from build123d import *

# Parameters (mm, degrees)
SKETCH2_R         = 104.775
SKETCH2_R_2       = 67.818
FLANGE_DEPTH      = 25.4
SKETCH4_R         = 81.407
SKETCH4_R_2       = 74.295
GROOVE_DEPTH      = 3.9878
SKETCH5_R         = 2.5527
SCREW_HOLES_DEPTH = 25.4
CIRPATTERN1_COUNT = 12


with BuildPart() as part:
    # Sketch2 → Flange (new body)
    with BuildSketch(Plane(origin=(0, 0, 0), x_dir=(1, 0, 0), z_dir=(0, 1, 0))):
        with Locations(Location((0, 0, 0), (0, 0, 270))):
            Circle(SKETCH2_R)
        with Locations(Location((0, 0, 0), (0, 0, 270))):
            Circle(SKETCH2_R_2, mode=Mode.SUBTRACT)
    extrude(amount=FLANGE_DEPTH)

    # Sketch4 → Groove (cut)
    with BuildSketch(Plane(origin=(0, 25.4, 0), x_dir=(1, 0, 0), z_dir=(0, 1, 0))):
        with Locations(Location((0, 0, 0), (0, 0, 270))):
            Circle(SKETCH4_R)
        with Locations(Location((0, 0, 0), (0, 0, 270))):
            Circle(SKETCH4_R_2, mode=Mode.SUBTRACT)
    extrude(amount=-GROOVE_DEPTH, mode=Mode.SUBTRACT)

    # Sketch5 → Screw Holes (cut)
    with BuildSketch(Plane(origin=(0, 25.4, 0), x_dir=(1, 0, 0), z_dir=(0, 1, 0))):
        with Locations(Location((0, -97.25025, 0), (0, 0, 270))):
            Circle(SKETCH5_R)
    screw_holes = extrude(amount=-SCREW_HOLES_DEPTH, mode=Mode.SUBTRACT)

    # CirPattern1: Screw Holes ×12 about axis
    cirpattern1_axis = Axis((0, 0, 0), (0, 1, 0))
    for i in range(1, CIRPATTERN1_COUNT):
        add(screw_holes.rotate(cirpattern1_axis, i * 360 / CIRPATTERN1_COUNT), mode=Mode.SUBTRACT)


solid = part.part
Geometry check sheet. Reference: the model listing, model coordinates, mm. A direction names the side the tool comes from. Round coordinates to 2 decimals unless told otherwise and drop trailing zeros. Write each loop counter-clockwise with the first axis right and the second up, starting at its lowest first coordinate (ties: lowest second). Pieces come first, ordered by that corner, then holes.
Item 1: Section check B-B (x = 0). Record the boundary of the cut face in (y, z) (3 decimals).
Determined:
outline: (0, -104.775) - (25.4, -104.775) - (25.4, -99.803) - (0, -99.803) - close; (0, -94.698) - (25.4, -94.698) - (25.4, -81.407) - (21.412, -81.407) - (21.412, -74.295) - (25.4, -74.295) - (25.4, -67.818) - (0, -67.818) - close; (0, 67.818) - (25.4, 67.818) - (25.4, 74.295) - (21.412, 74.295) - (21.412, 81.407) - (25.4, 81.407) - (25.4, 94.698) - (0, 94.698) - close; (0, 99.803) - (25.4, 99.803) - (25.4, 104.775) - (0, 104.775) - close
Item 2: Material ranges on line 1 along X through (y, z) = (17.75, -0.5); line 2 along Z through (x, y) = (-43, 24); line 3 along Z through (x, y) = (-50, 12), recorded low to high.
Determined:
line 1: x = -104.77 to -99.75, -94.75 to -67.82, 67.82 to 94.75, 99.75 to 104.77
line 2: z = -95.54 to -69.12, -60.59 to -52.44, 52.44 to 60.59, 69.12 to 95.54
line 3: z = -92.07 to -86.37, -82.07 to -45.82, 45.82 to 82.07, 86.37 to 92.07
Item 3: Mould release check, pull along X, two halves, no side actions. Record for faces 1 (the face through (82.5, 12.88, 50.51)), 2 (the face through (-62, 25.4, 54)), 3 (the face through (-102.283, 12.522, -22.713)): +X half, -X half, draft (parallel to the pull), parting line (faces both ways), or undercut.
Determined:
face 1: undercut
face 2: draft
face 3: parting line
Item 4: Section check C-C (z = 59.5). Record the boundary of the cut face in (x, y), plus the area to 3 significant figures.
Determined:
outline: (-86.24, 0) - (-32.54, 0) - (-32.54, 25.4) - (-44.49, 25.4) - (-44.49, 21.41) - (-55.56, 21.41) - (-55.56, 25.4) - (-86.24, 25.4) - close; (32.54, 0) - (86.24, 0) - (86.24, 25.4) - (55.56, 25.4) - (55.56, 21.41) - (44.49, 21.41) - (44.49, 25.4) - (32.54, 25.4) - close
area: 2,640 mm2
Item 5: Go/stop test with flat-tipped pins: pin 1 Ø1 at (y, z) = (13.5, -68.5) entering from +X; pin 2 Ø4 at (x, y) = (74.5, 12) entering from +Z; pin 3 Ø5 at (y, z) = (19.5, -64.5) entering from +X; pin 4 Ø3 at (x, z) = (-83.5, 68) entering from -Y. Record where each tip stops, or that it passes through.
Determined:
pin 1: stops at x = 79.71
pin 2: stops at z = 75.64
pin 3: stops at x = 84.46
pin 4: passes through
Item 6: Section check A-A (z = 0). Record the boundary of the cut face in (x, y) (3 decimals).
Determined:
outline: (-104.775, 0) - (-99.803, 0) - (-99.803, 25.4) - (-104.775, 25.4) - close; (-94.698, 0) - (-67.818, 0) - (-67.818, 25.4) - (-74.295, 25.4) - (-74.295, 21.412) - (-81.407, 21.412) - (-81.407, 25.4) - (-94.698, 25.4) - close; (67.818, 0) - (94.698, 0) - (94.698, 25.4) - (81.407, 25.4) - (81.407, 21.412) - (74.295, 21.412) - (74.295, 25.4) - (67.818, 25.4) - close; (99.803, 0) - (104.775, 0) - (104.775, 25.4) - (99.803, 25.4) - close
Item 7: Access from +Z, -Z, +X, -X, +Y, -Y to the whole of each face (thin tool, end or side, straight path). Record for faces 4 (the face through (-79.47, 23.43, -17.65)), 5 (the face through (-0.1, 12.9, -94.7)).
Determined:
face 4: +Y
face 5: +Y, -Y
Item 8: Section check D-D (x = 25.5). Record the boundary of the cut face in (y, z), plus the area to 3 significant figures.
Determined:
outline: (0, -101.62) - (25.4, -101.62) - (25.4, -77.31) - (21.41, -77.31) - (21.41, -69.78) - (25.4, -69.78) - (25.4, -62.84) - (0, -62.84) - close; (0, 62.84) - (25.4, 62.84) - (25.4, 69.78) - (21.41, 69.78) - (21.41, 77.31) - (25.4, 77.31) - (25.4, 101.62) - (0, 101.62) - close
area: 1,910 mm2
